The model under review builds one solid part; all positions refer to its coordinate system, in mm. Face numbers are marked on the shaded views. A direction names the side the tool comes from. Coordinates: 2 decimals unless noted, no trailing zeros. Order: outer loops, then holes, each group sorted by start corner. A loop starts at its lowest first (then second) coordinate and runs counter-clockwise, first axis right, second up. Notation, with made-up numbers: (29, 89) -> (82, 89) arc R10 cw to (82, 105) -> close; hole circle Ø8 at (70.25, 6). An arc over 180 degrees is marked (long way). Use one line per item in the form item = value.
from build123d import *

# Parameters (mm, degrees)
SKETCH_1_W           = 34
SKETCH_1_H           = 20
EXTRUDE_1_DEPTH      = 30
SKETCH_2_W           = 29
SKETCH_2_H           = 20
CUT_EXTRUDE_1_DEPTH  = 25
SKETCH_7_R           = 9.5
EXTRUDE_3_DEPTH      = 4
SKETCH_4_R           = 1.5
CUT_EXTRUDE_5_DEPTH  = 5
SKETCH_6_R           = 9.5
EXTRUDE_2_DEPTH      = 4
SKETCH_5_R           = 1.5
CUT_EXTRUDE_6_DEPTH  = 10
SKETCH_9_R           = 3
CUT_EXTRUDE_7_DEPTH  = 10
SKETCH_10_R          = 3
CUT_EXTRUDE_8_DEPTH  = 10
EXTRUDE_4_DEPTH      = 2
EXTRUDE_5_DEPTH      = 2
SKETCH_14_W          = 5
SKETCH_14_H          = 24
EXTRUDE_6_DEPTH      = 2
SKETCH_15_W          = 5
SKETCH_15_H          = 24
EXTRUDE_7_DEPTH      = 2
SKETCH_16_R          = 3
CUT_EXTRUDE_10_DEPTH = 4
SKETCH_17_R          = 3
CUT_EXTRUDE_11_DEPTH = 4
FILLET_5_R           = 10
FILLET_6_R           = 10
FILLET_9_R           = 10
FILLET_10_R          = 10
FILLET_11_R          = 5
FILLET_12_R          = 2
FILLET_13_R          = 2
FILLET_14_R          = 2


with BuildPart() as part:
    # 草图1 → 凸台-拉伸1 (new body)
    with BuildSketch(Plane.XY):
        with Locations((4.298701299, 4.025974026)):
            Rectangle(SKETCH_1_W, SKETCH_1_H)
    extrude(amount=EXTRUDE_1_DEPTH)

    # 草图2 → 切除-拉伸1 (cut)
    with BuildSketch(Plane(origin=(0, 0, 0), x_dir=(-1, 0, 0), z_dir=(0, 0, -1))):
        with Locations((-6.798701299, 4.025974026)):
            Rectangle(SKETCH_2_W, SKETCH_2_H)
    extrude(amount=-CUT_EXTRUDE_1_DEPTH, mode=Mode.SUBTRACT)

    # 草图7 → 凸台-拉伸3 (add)
    with BuildSketch(Plane.ZY.offset(12.701298701)):
        with Locations((10, 4.025974026)):
            Circle(SKETCH_7_R)
    extrude(amount=EXTRUDE_3_DEPTH)

    # 草图4 → 切除-拉伸5 (cut, symmetric)
    with BuildSketch(Plane.ZY.offset(12.701298701)):
        with Locations((10, 11.025974026)):
            Circle(SKETCH_4_R)
        with Locations((3, 4.025974026)):
            Circle(SKETCH_4_R)
        with Locations((10, -2.974025974)):
            Circle(SKETCH_4_R)
        with Locations((17, 4.025974026)):
            Circle(SKETCH_4_R)
    extrude(amount=CUT_EXTRUDE_5_DEPTH, both=True, mode=Mode.SUBTRACT)

    # 草图6 → 凸台-拉伸2 (add)
    with BuildSketch(Plane(origin=(0, 0, 25), x_dir=(-1, 0, 0), z_dir=(0, 0, -1))):
        with Locations((-11.298701299, 4.025974026)):
            Circle(SKETCH_6_R)
    extrude(amount=EXTRUDE_2_DEPTH)

    # 草图5 → 切除-拉伸6 (cut)
    with BuildSketch(Plane.XY.offset(30)):
        with Locations((11.298701299, 11.025974026)):
            Circle(SKETCH_5_R)
        with Locations((11.298701299, -2.974025974)):
            Circle(SKETCH_5_R)
        with Locations((4.298701299, 4.025974026)):
            Circle(SKETCH_5_R)
        with Locations((18.298701299, 4.025974026)):
            Circle(SKETCH_5_R)
    extrude(amount=-CUT_EXTRUDE_6_DEPTH, mode=Mode.SUBTRACT)

    # 草图9 → 切除-拉伸7 (cut)
    with BuildSketch(Plane(origin=(0, 0, 21), x_dir=(-1, 0, 0), z_dir=(0, 0, -1))):
        with Locations((-11.298701299, 4.025974026)):
            Circle(SKETCH_9_R)
    extrude(amount=-CUT_EXTRUDE_7_DEPTH, mode=Mode.SUBTRACT)

    # 草图10 → 切除-拉伸8 (cut)
    with BuildSketch(Plane.ZY.offset(16.701298701)):
        with Locations((10, 4.025974026)):
            Circle(SKETCH_10_R)
    extrude(amount=-CUT_EXTRUDE_8_DEPTH, mode=Mode.SUBTRACT)

    # 草图12 → 凸台-拉伸4 (add)
    with BuildSketch(Plane(origin=(0, 14.025974026, 0), x_dir=(1, 0, 0), z_dir=(0, 1, 0))):
        Polygon((21.298701299, -25), (-7.701298701, -25), (-7.701298701, 0), (-12.701298701, 0), (-12.701298701, -30), (21.298701299, -30), align=None)
    extrude(amount=EXTRUDE_4_DEPTH)

    # 草图13 → 凸台-拉伸5 (add)
    with BuildSketch(Plane.XZ.offset(5.974025974)):
        Polygon((-7.701298701, 25), (21.298701299, 25), (21.298701299, 30), (-12.701298701, 30), (-12.701298701, 0), (-7.701298701, 0), align=None)
    extrude(amount=EXTRUDE_5_DEPTH)

    # 草图14 → 凸台-拉伸6 (add)
    with BuildSketch(Plane(origin=(21.298701299, 0, 0), x_dir=(0, 0, -1), z_dir=(1, 0, 0))):
        with Locations((-27.5, 4.025974026)):
            Rectangle(SKETCH_14_W, SKETCH_14_H)
    extrude(amount=EXTRUDE_6_DEPTH)

    # 草图15 → 凸台-拉伸7 (add)
    with BuildSketch(Plane(origin=(0, 0, 0), x_dir=(-1, 0, 0), z_dir=(0, 0, -1))):
        with Locations((10.201298701, 4.025974026)):
            Rectangle(SKETCH_15_W, SKETCH_15_H)
    extrude(amount=EXTRUDE_7_DEPTH)

    # 草图16 → 切除-拉伸10 (cut)
    with BuildSketch(Plane.XY.offset(30)):
        with Locations((11.298701299, 11.025974026)):
            Circle(SKETCH_16_R)
        with Locations((4.298701299, 4.025974026)):
            Circle(SKETCH_16_R)
        with Locations((11.298701299, -2.974025974)):
            Circle(SKETCH_16_R)
        with Locations((18.298701299, 4.025974026)):
            Circle(SKETCH_16_R)
    extrude(amount=-CUT_EXTRUDE_10_DEPTH, mode=Mode.SUBTRACT)

    # 草图17 → 切除-拉伸11 (cut)
    with BuildSketch(Plane(origin=(-7.701298701, 0, 0), x_dir=(0, 0, -1), z_dir=(1, 0, 0))):
        with Locations(Location((-10, 11.025974026, 0), (0, 0, 90))):
            Circle(SKETCH_17_R)
        with Locations(Location((-17, 4.025974026, 0), (0, 0, 90))):
            Circle(SKETCH_17_R)
        with Locations(Location((-10, -2.974025974, 0), (0, 0, 90))):
            Circle(SKETCH_17_R)
        with Locations(Location((-3, 4.025974026, 0), (0, 0, 90))):
            Circle(SKETCH_17_R)
    extrude(amount=-CUT_EXTRUDE_11_DEPTH, mode=Mode.SUBTRACT)

    # 圆角5
    fillet_5_edges = [part.edges().sort_by_distance(p)[0] for p in [
        (-10.201298701, 16.025974026, -2),
    ]]
    fillet(fillet_5_edges, radius=FILLET_5_R)

    # 圆角6
    fillet_6_edges = [part.edges().sort_by_distance(p)[0] for p in [
        (-10.201298701, -7.974025974, -2),
    ]]
    fillet(fillet_6_edges, radius=FILLET_6_R)

    # 圆角9
    fillet_9_edges = [part.edges().sort_by_distance(p)[0] for p in [
        (23.298701299, -7.974025974, 27.5),
    ]]
    fillet(fillet_9_edges, radius=FILLET_9_R)

    # 圆角10
    fillet_10_edges = [part.edges().sort_by_distance(p)[0] for p in [
        (23.298701299, 16.025974026, 27.5),
    ]]
    fillet(fillet_10_edges, radius=FILLET_10_R)

    # 圆角11
    fillet_11_edges = [part.edges().sort_by_distance(p)[0] for p in [
        (-12.701298701, 4.025974026, 30),
    ]]
    fillet(fillet_11_edges, radius=FILLET_11_R)

    # 圆角12
    fillet_12_edges = [part.edges().sort_by_distance(p)[0] for p in [
        (-12.701298701, 16.025974026, 16.5),
        (-12.701298701, 13.097041838, 0.928932188),
        (-12.701298701, 4.025974026, -2),
        (-12.701298701, -5.045093786, 0.928932188),
        (2.798701299, -7.974025974, 30),
        (20.369769111, -5.045093786, 30),
        (23.298701299, 4.025974026, 30),
        (20.369769111, 13.097041838, 30),
        (2.798701299, 16.025974026, 30),
        (-12.701298701, -7.974025974, 16.5),
        (-11.236832607, -7.974025974, 28.535533906),
        (-11.236832607, 16.025974026, 28.535533906),
    ]]
    fillet(fillet_12_edges, radius=FILLET_12_R - 0.0001)  # a hair under: the kernel refuses the full size

    # 圆角13
    fillet_13_edges = [part.edges().sort_by_distance(p)[0] for p in [
        (2.798701299, -7.974025974, 25),
        (23.298701299, 4.025974026, 25),
        (20.369769111, -5.045093786, 25),
        (2.798701299, 16.025974026, 25),
        (20.369769111, 13.097041838, 25),
    ]]
    fillet(fillet_13_edges, radius=FILLET_13_R)

    # 圆角14
    fillet_14_edges = [part.edges().sort_by_distance(p)[0] for p in [
        (-7.701298701, 16.025974026, 17.5),
        (-7.701298701, 13.097041838, 0.928932188),
        (-7.701298701, 4.025974026, -2),
        (-7.701298701, -5.045093786, 0.928932188),
        (-7.701298701, -7.974025974, 17.5),
    ]]
    fillet(fillet_14_edges, radius=FILLET_14_R - 0.0001)  # a hair under: the kernel refuses the full size


solid = part.part
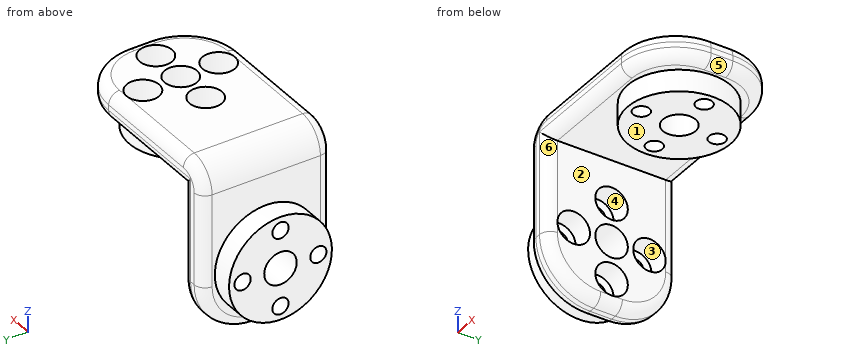
Item 1: To check wall thickness, follow L1, parallel to Z at x = -10.5, y = 1.5; L2, parallel to X at y = 10.75, z = 22; L3, parallel to Z at x = -13, y = -2.5. State the ranges of each line that lie inside material, in increasing order. Write a range as from..to.
Results found:
L1 = -1.99..1.38, 4.62..8.38, 11.62..15.38, 18.62..29.14
L2 = -12.7..-7.7, 4.59..9.82, 12.77..18.01
L3 = 3.1..8.58, 11.42..16.9
Item 2: We need section B-B (z = 17.5). Write out the cut boundary in (x, y).
Results found:
outline = (-16.7, -1.8) -> (-12.7, -1.8) -> (-12.7, -5.97) arc R2 ccw to (-10.7, -7.97) -> (-9.7, -7.97) arc R2 ccw to (-7.7, -5.97) -> (-7.7, 1.07) -> (-11.7, 1.07) -> (-11.7, 2.61) -> (-16.7, 2.61) -> close; (-16.7, 5.44) -> (-11.7, 5.44) -> (-11.7, 6.98) -> (-7.7, 6.98) -> (-7.7, 14.03) arc R2 ccw to (-9.7, 16.03) -> (-10.7, 16.03) arc R2 ccw to (-12.7, 14.03) -> (-12.7, 9.86) -> (-16.7, 9.86) -> close
Item 3: Draft analysis for pull direction Y (two halves, no side actions). For the marked faces 4, 5 and 6, state which applies: released by +Y, released by -Y, zero draft, split by the parting line, or undercut.
Results found:
face_4 = undercut
face_5 = zero draft
face_6 = released by -Y
Item 4: We need section C-C (z = 10). State how many separate pieces and enclosed holes the cut face has, plus the area to 3 significant figures.
Results found:
separate_pieces = 4
enclosed_holes = 0
area = 60.6 mm²
Item 5: Clearance check with flat-ended pins moving along their axes: pin 1 (6 mm diameter, centred on x = 9, y = 1, fed in from -Z); pin 2 (7 mm diameter, centred on y = 4.03, z = 10, fed in from -X); pin 3 (3 mm diameter, centred on x = 18.5, y = 3, fed in from +Z); pin 4 (5 mm diameter, centred on x = -5, z = 19.5, fed in from +Y). State where each tip first meets the part, or that it passes through.
Results found:
pin_1 = 21
pin_2 = -16.7
pin_3 = 26
pin_4 = through
Item 6: We need section D-D (z = 24). Write out the cut boundary in (x, y).
Results found:
outline = (-12.7, -5.97) arc R2 ccw to (-10.7, -7.97) -> (-9.7, -7.97) arc R2 ccw to (-7.7, -5.97) -> (-7.7, 14.03) arc R2 ccw to (-9.7, 16.03) -> (-10.7, 16.03) arc R2 ccw to (-12.7, 14.03) -> close; circle Ø19 at (11.3, 4.03); hole circle Ø3 at (4.3, 4.03); hole circle Ø6 at (11.3, 4.03); hole circle Ø3 at (11.3, -2.97); hole circle Ø3 at (11.3, 11.03); hole circle Ø3 at (18.3, 4.03)
Item 7: Tool access review of the marked faces 1, 2 and 3: name each direction out of +Z, -Z, +X, -X, +Y, -Y from which nothing blocks a thin tool from reaching the whole face with its end or side.
Results found:
face_1 = -Z, +X, +Y, -Y
face_2 = -Z, +Y, -Y
face_3 = +X
Item 8: We need section A-A (x = 0). Write out the cut boundary in (y, z).
Results found:
outline = (-7.97, 27) arc R2 ccw to (-5.97, 25) -> (14.03, 25) arc R2 ccw to (16.03, 27) -> (16.03, 28) arc R2 ccw to (14.03, 30) -> (-5.97, 30) arc R2 ccw to (-7.97, 28) -> close
